Here's the drawing with two shaded views (mm, measured from the low corner). I have some questions. Round coordinates to 2 decimals unless told otherwise and drop trailing zeros. Order: outer loops, then holes, each group sorted by start corner. A loop starts at its lowest first (then second) coordinate and runs counter-clockwise, first axis right, second up.
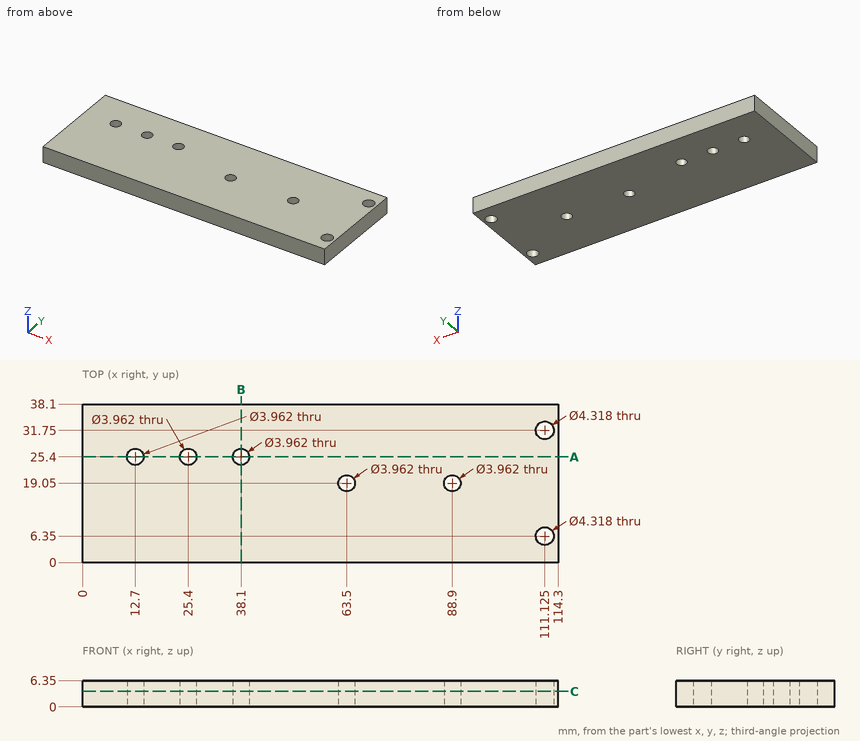
1. I need wall thicknesses on probe 1 along X at (y, z) = (25.4, 3.25); probe 2 along Y at (x, z) = (63.5, 2); probe 3 along Y at (x, z) = (38, 3.75). Which ranges of each line are inside material? Lowest first, please.
Evaluation:
probe 1: x = 0 to 10.72, 14.68 to 23.42, 27.38 to 36.12, 40.08 to 114.3
probe 2: y = 0 to 17.07, 21.03 to 38.1
probe 3: y = 0 to 23.42, 27.38 to 38.1
2. If we section it at A-A, the plane y = 25.4: Write out the boundary of the cut face in (x, z).
Evaluation:
outline: (0, 0) - (10.72, 0) - (10.72, 6.35) - (0, 6.35) - close; (14.68, 0) - (23.42, 0) - (23.42, 6.35) - (14.68, 6.35) - close; (27.38, 0) - (36.12, 0) - (36.12, 6.35) - (27.38, 6.35) - close; (40.08, 0) - (114.3, 0) - (114.3, 6.35) - (40.08, 6.35) - close
3. If we section it at C-C, the plane z = 3.75: State how many separate pieces and enclosed holes the cut face has, and give its area (3 significant figures).
Evaluation:
separate pieces: 1
enclosed holes: 7
area: 4,260 mm2
4. I'm going to push a flat-ended pin straight in: P1, Ø3.5, axis at x = 88.9, y = 19.05, coming from the +Z side. Where does the tip first touch, or does it pass through?
Evaluation:
P1: passes through
5. If we section it at B-B, the plane x = 38.1: Write out the boundary of the cut face in (y, z), and give its area (3 significant figures).
Evaluation:
outline: (0, 0) - (23.42, 0) - (23.42, 6.35) - (0, 6.35) - close; (27.38, 0) - (38.1, 0) - (38.1, 6.35) - (27.38, 6.35) - close
area: 217 mm2
